from build123d import *

# Parameters (mm, degrees)
BOX005_W        = 58
BOX005_H        = 110
BOX005_DEPTH    = 1.5
FILLET002_R     = 5
SKETCH008_R     = 1.5
POCKET003_DEPTH = 5


with BuildPart() as part:
    # Box005 → Box005 (new body)
    with BuildSketch(Plane(origin=(-2, -13, -1.5), x_dir=(1, 0, 0), z_dir=(0, 0, 1))):
        with Locations((29, 55)):
            Rectangle(BOX005_W, BOX005_H)
    extrude(amount=BOX005_DEPTH)

    # Fillet002
    fillet002_edges = [part.edges().sort_by_distance(p)[0] for p in [
        (-2, -13, -0.75),
        (-2, 97, -0.75),
        (56, -13, -0.75),
        (56, 97, -0.75),
    ]]
    fillet(fillet002_edges, radius=FILLET002_R)

    # Sketch008 → Pocket003 (cut)
    with BuildSketch(Plane.XY):
        with Locations((3, 92)):
            Circle(SKETCH008_R)
        with Locations((51, 92)):
            Circle(SKETCH008_R)
        with Locations((3, -8)):
            Circle(SKETCH008_R)
        with Locations((51, -8)):
            Circle(SKETCH008_R)
    extrude(amount=-POCKET003_DEPTH, mode=Mode.SUBTRACT)


solid = part.part
The model under review builds one solid part; all positions refer to its coordinate system, in mm. Give positions to 0.01 mm unless a question says otherwise; leave off trailing zeros. One line per question, with ' | ' between items. Start each with the question number.
1) Wall thickness on L1, parallel to X at y = 92, z = -0.8; L2, parallel to Y at x = 51, z = -1: over which ranges is each line inside the solid? List them lowest first. Write a range as from..to.
2) Mouldability with a two-part tool opening along Y and no side actions: class faces 1 (the face through (50.805, 93.487, -0.74)), 2 (the face through (54, -12, -1)), 3 (the face through (-1, 95, -1)) as pulls with the +Y half, pulls with the -Y half, needs draft (parallel to the pull), parting line crosses it, or undercut.
3) Clearance check with a flat-ended pin moving along its axis: P1, Ø1.8, axis at x = 51, y = 92, coming from the -Z side. State where the tip first meets the part, or that it passes through.
Found:
1) L1: x = -2..1.5, 4.5..49.5, 52.5..56 | L2: y = -13..-9.5, -6.5..90.5, 93.5..97
2) face 1: undercut | face 2: pulls with the -Y half | face 3: pulls with the +Y half
3) P1: passes through
